```python
from build123d import *

# Parameters (mm, degrees)
SKETCH1_R           = 9
BOSS_EXTRUDE1_DEPTH = 12
SKETCH1_3_R         = 6
BOSS_EXTRUDE2_DEPTH = 32
CUT_EXTRUDE1_DEPTH  = 6


with BuildPart() as part:
    # Sketch1 → Boss-Extrude1 (new body)
    with BuildSketch(Plane(origin=(0, 0, 0), x_dir=(1, 0, 0), z_dir=(0, 1, 0))):
        with Locations(Location((0, 0, 0), (0, 0, 270))):
            Circle(SKETCH1_R)
    extrude(amount=BOSS_EXTRUDE1_DEPTH)

    # Sketch1_3 → Boss-Extrude2 (add)
    with BuildSketch(Plane(origin=(0, 0, 0), x_dir=(1, 0, 0), z_dir=(0, 1, 0))):
        with Locations(Location((0, 0, 0), (0, 0, 270))):
            Circle(SKETCH1_3_R)
    extrude(amount=BOSS_EXTRUDE2_DEPTH)

    # Sketch2 → Cut-Extrude1 (cut)
    with BuildSketch(Plane.XZ):
        Polygon((-3.5, -6.062177826), (3.5, -6.062177826), (7, 0), (3.5, 6.062177826), (-3.5, 6.062177826), (-7, 0), align=None)
    extrude(amount=-CUT_EXTRUDE1_DEPTH, mode=Mode.SUBTRACT)


solid = part.part
```
The listing builds one solid part. Answer for the finished solid, in the listing's coordinates (mm). A direction names the side the tool comes from. Round coordinates to 2 decimals unless told otherwise and drop trailing zeros. Write each loop counter-clockwise with the first axis right and the second up, starting at its lowest first coordinate (ties: lowest second). Pieces come first, ordered by that corner, then holes. Notation, with made-up numbers: (56, 17.25) -> (65, 17.25) arc R20 ccw to (65, 40.25) -> close; hole circle Ø1 at (46.5, 13). An arc over 180 degrees is marked (long way). Answer as a JSON object with one key per item and string values. Group by question number.
Q1. Section D-D (z = -7.5) is taken. Write down the section's boundary in (x, y), plus the area to 3 significant figures.
Q2. Section B-B (z = 1) is taken. Write down the section's boundary in (x, y).
Q3. Straight lines are drawn through the part: line 1 along Y through (x, z) = (-2.5, -0.5); line 2 along Y through (x, z) = (-8, 1.75); line 3 along X through (y, z) = (2.5, 5.25). For each, find the intervals that lie inside material, in ascending order.
Q4. Section C-C (y = 16) is taken. Write down the section's boundary in (x, z).
Q5. Determine the mould class of faces 4 (the face through (-5.226, 2.958, 3.074)), 5 (the face through (2.703, 5.916, 8.584)), 6 (the face through (0, 32, 0)), 7 (the face through (0, 3, -6.062)) for opening direction X: pulls with the +X half, pulls with the -X half, needs draft (parallel to the pull), parting line crosses it, or undercut.
Q6. Section A-A (x = 0) is taken. Write down the section's boundary in (y, z).
Q7. Each of these flat-tipped pins is pushed along its axis until it touches: pin 1 Ø2 at (x, y) = (2.5, 9) entering from +Z; pin 2 Ø3 at (x, y) = (3.5, 7) entering from +Z; pin 3 Ø6 at (x, z) = (-0.5, -1) entering from -Y. Where does it stop, or does it pass through?
Q8. Which of the six approach directions +Z, -Z, +X, -X, +Y, -Y give full straight-line access (tool end or side, diameter ignored) to faces 1 (the face through (6.1, 0, -2.1)), 2 (the face through (5.274, 2.958, 2.989)), 3 (the face through (1.802, 21.86, 5.723))?
Check values:
{
 "1": {"outline": "(-4.97, 0) -> (4.97, 0) -> (4.97, 12) -> (-4.97, 12) -> close", "area": "119 mm^2"},
 "2": {"outline": "(-8.94, 0) -> (-6.42, 0) -> (-6.42, 6) -> (6.42, 6) -> (6.42, 0) -> (8.94, 0) -> (8.94, 12) -> (5.92, 12) -> (5.92, 32) -> (-5.92, 32) -> (-5.92, 12) -> (-8.94, 12) -> close"},
 "3": {"line 1": "6 to 32", "line 2": "0 to 12", "line 3": "-7.31 to -3.97, 3.97 to 7.31"},
 "4": {"outline": "circle Ø12 at (0, 0)"},
 "5": {"face 4": "undercut", "face 5": "parting line crosses it", "face 6": "needs draft", "face 7": "undercut"},
 "6": {"outline": "(0, -9) -> (12, -9) -> (12, -6) -> (32, -6) -> (32, 6) -> (12, 6) -> (12, 9) -> (0, 9) -> (0, 6.06) -> (6, 6.06) -> (6, -6.06) -> (0, -6.06) -> close"},
 "7": {"pin 1": "z = 8.87", "pin 2": "z = 8.77", "pin 3": "y = 6"},
 "8": {"face 1": "+Z, -Z, +X, -X, -Y", "face 2": "-Y", "face 3": "+Y"}
}
